Model file for the job. Use its own axes, mm. A direction names the side the tool comes from. Round coordinates to 2 decimals unless told otherwise and drop trailing zeros. Write each loop counter-clockwise with the first axis right and the second up, starting at its lowest first coordinate (ties: lowest second). Pieces come first, ordered by that corner, then holes. Notation, with made-up numbers: (37.25, -0.75) - (88.25, -0.75) arc R30 ccw to (88.25, 37.25) - close; hole circle Ø10 at (55.25, 46). An arc over 180 degrees is marked (long way). One line per item, written item: value.
from build123d import *

# Parameters (mm, degrees)
SKETCH1_W           = 5
SKETCH1_H           = 70
BOSS_EXTRUDE1_DEPTH = 3
SKETCH2_R           = 2.5
BOSS_EXTRUDE2_DEPTH = 20
SKETCH3_R           = 2.5
BOSS_EXTRUDE3_DEPTH = 20
SKETCH4_R           = 1.5
CUT_EXTRUDE1_DEPTH  = 20


with BuildPart() as part:
    # Sketch1 → Boss-Extrude1 (new body)
    with BuildSketch(Plane.XY):
        with Locations((2.5, 35)):
            Rectangle(SKETCH1_W, SKETCH1_H)
    extrude(amount=BOSS_EXTRUDE1_DEPTH)

    # Sketch2 → Boss-Extrude2 (add)
    with BuildSketch(Plane.XY.offset(3)):
        with Locations((2.5, 2.5)):
            Circle(SKETCH2_R)
    extrude(amount=BOSS_EXTRUDE2_DEPTH)

    # Sketch3 → Boss-Extrude3 (add)
    with BuildSketch(Plane(origin=(0, 0, 0), x_dir=(-1, 0, 0), z_dir=(0, 0, -1))):
        with Locations((-2.5, 40)):
            Circle(SKETCH3_R)
    extrude(amount=BOSS_EXTRUDE3_DEPTH)

    # Sketch4 → Cut-Extrude1 (cut)
    with BuildSketch(Plane(origin=(0, 0, 0), x_dir=(-1, 0, 0), z_dir=(0, 0, -1))):
        with Locations((-2.5, 67.5)):
            Circle(SKETCH4_R)
    extrude(amount=-CUT_EXTRUDE1_DEPTH, mode=Mode.SUBTRACT)


solid = part.part
1. Wall check: probe 1 along Y at (x, z) = (2.5, 2.2); probe 2 along X at (y, z) = (67.5, 0.8); probe 3 along Z at (x, y) = (1.4, 35). Give the ranges that are in metal, low to high. Write a range as [from, to].
Report:
probe 1: [0, 66], [69, 70]
probe 2: [0, 1], [4, 5]
probe 3: [0, 3]
2. Band-saw the part on C-C on z = -13.5. Write the cut outline in (x, y).
Report:
outline: circle Ø5 at (2.5, 40)
3. Band-saw the part on D-D on y = 18. Write the cut outline in (x, z).
Report:
outline: (0, 0) - (5, 0) - (5, 3) - (0, 3) - close
4. Band-saw the part on A-A on y = 67.5. Write the cut outline in (x, z), plus the area to 3 significant figures.
Report:
outline: (0, 0) - (1, 0) - (1, 3) - (0, 3) - close; (4, 0) - (5, 0) - (5, 3) - (4, 3) - close
area: 6.00 mm²
5. Mould opens along Y. For faces 1 (the face through (1.694, 68.765, 1.479)), 2 (the face through (2, 70, 1)), 3 (the face through (0.5, 1, 12.9)), 4 (the face through (5, 35, 1)) say: released by +Y, released by -Y, zero draft, split by the parting line, or undercut.
Report:
face 1: undercut
face 2: released by +Y
face 3: split by the parting line
face 4: zero draft
6. Tool access for faces 5 (the face through (4.5, 0.5, 3)), 6 (the face through (2, 0, 1)), 7 (the face through (0.5, 0.6, 3)), 8 (the face through (3.04, 37.56, -9.86)), 9 (the face through (3, 40, -20)): list every direction of +Z, -Z, +X, -X, +Y, -Y with a clear straight run to the whole face (end or side of a thin tool).
Report:
face 5: +Z, +X, -Y
face 6: +Z, -Z, +X, -X, -Y
face 7: +Z, -X, -Y
face 8: -Z
face 9: -Z, +X, -X, +Y, -Y
7. Drop flat-ended pins along their axis: pin 1 (2.5 mm diameter, centred on x = 1.5, y = 45, fed in from +Z); pin 2 (1.5 mm diameter, centred on x = 2.5, y = 23.5, fed in from -Z); pin 3 (10 mm diameter, centred on y = 44.5, z = -12.5, fed in from +X). Give the stop position or say it passes through.
Report:
pin 1: z = 3
pin 2: z = 0
pin 3: x = 5
8. Band-saw the part on B-B on y = 38.5. Write the cut outline in (x, z), plus the area to 3 significant figures.
Report:
outline: (0, 0) - (0.5, 0) - (0.5, -20) - (4.5, -20) - (4.5, 0) - (5, 0) - (5, 3) - (0, 3) - close
area: 95.0 mm²
